Part model, mm, in its own coordinate system. A direction names the side the tool comes from. Round coordinates to 2 decimals unless told otherwise and drop trailing zeros. Write each loop counter-clockwise with the first axis right and the second up, starting at its lowest first coordinate (ties: lowest second). Pieces come first, ordered by that corner, then holes. Notation, with made-up numbers: (72.5, 68) -> (110.5, 68) arc R20 cw to (110.5, 93) -> close; hole circle Ø5 at (86, 8.25). An arc over 180 degrees is marked (long way). Use CSV: the item, a comma, the result in double quotes. Start each with the question number.
(1) Two-plate mould, pull along X, no slides. Class faces 1 (the flat face through (28, -14.05, -3)), 2 (the flat face through (21, 0, 6.5)), 3 (the flat face through (19.117, -16.704, 2.958)), 4 (the flat face through (29.408, -13, -1)): released by +X, released by -X, zero draft, split by the parting line, or undercut.
(2) Saw through at C-C (x = 10.5). Give the cut face in (y, z).
(3) Drop flat-ended pins along their axis: pin 1 (1.3 mm diameter, centred on x = 8, y = -17.5, fed in from -Z); pin 2 (1.9 mm diameter, centred on y = -22.5, z = 1.5, fed in from -X); pin 3 (0.6 mm diameter, centred on x = -26, z = -2.5, fed in from +Y); pin 4 (1.6 mm diameter, centred on y = 15, z = -1, fed in from +X). Give the stop position or say it passes through.
(4) Saw through at B-B (z = 1.25). Count the separate pieces of the cut face and the enclosed holes in it, plus the area to 3 significant figures.
(5) Saw through at A-A (y = 0). Give the cut face in (x, z), plus the area to 3 significant figures.
(6) Probe line 1 (Y direction, x = -23, z = 0.75); line 2 (X direction, y = 19.79, z = 4.75) (3 decimals); line 3 (Y direction, x = 12, z = 6.25). List the from-to ranges inside material, lowest first. Write a range as [from, to].
(7) Which spindle directions (+Z, -Z, +X, -X, +Y, -Y) get a long thin tool onto all of the face, cutting with end or side? Do faces 5 (the flat face through (24.908, 0, 3)), 6 (the flat face through (-5, -23, 2)), 7 (the cylindrical face through (-25.1, -13, -2.7)), 8 (the cylindrical face through (8.29, -16.61, 5.01)). Say none if no direction does.
```python
from build123d import *

# Parameters (mm, degrees)
PAD_DEPTH       = 6.5
POCKET_DEPTH    = 6
SKETCH002_R     = 13.5
POCKET001_DEPTH = 1
SKETCH003_W     = 5.4
SKETCH003_H     = 6.5
PAD001_DEPTH    = 4.5
POCKET002_DEPTH = 10
SKETCH010_W     = 3.95
SKETCH010_H     = 6.5
PAD002_DEPTH    = 4.5
POCKET005_DEPTH = 10
SKETCH014_R     = 20.45
SKETCH014_R_2   = 19.5
POCKET008_DEPTH = 0.3
SKETCH015_R     = 2.2
SKETCH015_R_2   = 0.975
PAD003_DEPTH    = 2
POCKET009_DEPTH = 4
POCKET010_DEPTH = 4
PAD004_DEPTH    = 4
SKETCH019_R     = 0.6
POCKET011_DEPTH = 2
SKETCH020_R     = 0.6
POCKET012_DEPTH = 2
FILLET_R        = 4
CHAMFER_SIZE    = 2.5
FILLET001_R     = 5


with BuildPart() as part:
    # Sketch → Pad (new body)
    with BuildSketch(Plane.XY):
        with BuildLine():
            Line((-22.5019915649, 16), (-22.5019915649, -16))
            Line((-22.5019915649, -16), (-16.2858834577, -17.9000000001))
            ThreePointArc((-16.2858834577, -17.9000000001), (0.2206895737, -24.1989937004), (16.6096357576, -17.5999999999))
            Line((16.6096357576, -17.5999999999), (24.9082802252, -17.45))
            Line((24.9082802252, 17.45), (24.9082802252, -17.45))
            Line((16.6096357576, 17.6), (24.9082802252, 17.45))
            ThreePointArc((16.6096357576, 17.6), (0.2206895736, 24.1989937004), (-16.2858834578, 17.9))
            Line((-22.5019915649, 16), (-16.2858834578, 17.9))
        make_face()
    extrude(amount=PAD_DEPTH)

    # Sketch001 → Pocket (cut)
    with BuildSketch(Plane.XY):
        with BuildLine():
            Line((-14.8539557021, 16.9), (-21.2122180433, 15.55))
            Line((-21.2122180433, 15.55), (-21.2122180433, -15.55))
            Line((-21.2122180433, -15.55), (-14.8539557021, -16.9))
            ThreePointArc((-14.8539557021, -16.9), (-0.0760301383, -22.4998715423), (14.739402973, -17))
            Line((14.739402973, -17), (23.6191552218, -16.4))
            Line((23.6191552218, 16.4), (23.6191552218, -16.4))
            Line((14.739402973, 17), (23.6191552218, 16.4))
            ThreePointArc((14.739402973, 17), (-0.0760301383, 22.4998715423), (-14.8539557021, 16.9))
        make_face()
    extrude(amount=POCKET_DEPTH, mode=Mode.SUBTRACT)

    # Sketch002 (on Face19 of Pocket) → Pocket001 (cut)
    with BuildSketch(Plane(origin=(0, 0, 6), x_dir=(1, 0, 0), z_dir=(0, 0, -1))):
        Circle(SKETCH002_R)
    extrude(amount=-POCKET001_DEPTH, mode=Mode.SUBTRACT)

    # Sketch003 (on Face7 of Pad) → Pad001 (join)
    with BuildSketch(Plane.YZ.offset(24.9082802252)):
        with Locations((-14.75, 3.25)):
            Rectangle(SKETCH003_W, SKETCH003_H)
        with Locations((14.75, 3.25)):
            Rectangle(SKETCH003_W, SKETCH003_H)
    extrude(amount=PAD001_DEPTH)

    # Sketch006 (on Face22 of Pad001) → Pocket002 (cut)
    with BuildSketch(Plane.XY.offset(6.5)):
        with BuildLine():
            ThreePointArc((24.9082802252, 17.45), (26.9423471239, 15.7065020586), (29.4082802252, 14.6594169811))
            Line((29.4082802252, 17.45), (29.4082802252, 14.6594169811))
            Line((29.4082802252, 17.45), (24.9082802252, 17.45))
        make_face()
        with BuildLine():
            ThreePointArc((29.4082802252, -14.6594169811), (26.9423471239, -15.7065020586), (24.9082802252, -17.45))
            Line((29.4082802252, -17.45), (24.9082802252, -17.45))
            Line((29.4082802252, -14.6594169811), (29.4082802252, -17.45))
        make_face()
    extrude(amount=-POCKET002_DEPTH, mode=Mode.SUBTRACT)

    # Sketch010 (on Face3 of Pad) → Pad002 (join)
    with BuildSketch(Plane(origin=(-22.5019915649, 0, 0), x_dir=(0, -1, 0), z_dir=(-1, 0, 0))):
        with Locations((-14.025, 3.25)):
            Rectangle(SKETCH010_W, SKETCH010_H)
        with Locations((14.025, 3.25)):
            Rectangle(SKETCH010_W, SKETCH010_H)
    extrude(amount=PAD002_DEPTH)

    # Sketch011 (on Face28 of Pad002) → Pocket005 (cut)
    with BuildSketch(Plane.XY.offset(6.5)):
        Polygon((-27.0019915649, 16), (-22.5019915649, 16), (-27.0019915649, 14.5), align=None)
        Polygon((-22.5019915649, -16), (-27.0019915649, -14.5), (-27.0019915649, -16), align=None)
    extrude(amount=-POCKET005_DEPTH, mode=Mode.SUBTRACT)

    # Sketch014 (on Face10 of Pad) → Pocket008 (cut)
    with BuildSketch(Plane.XY.offset(6.5)):
        Circle(SKETCH014_R)
        Circle(SKETCH014_R_2, mode=Mode.SUBTRACT)
    extrude(amount=-POCKET008_DEPTH, mode=Mode.SUBTRACT)

    # Sketch015 (on Face19 of Pocket) → Pad003 (join)
    with BuildSketch(Plane(origin=(0, 0, 6), x_dir=(1, 0, 0), z_dir=(0, 0, -1))):
        with Locations((-18.42, 13.32)):
            Circle(SKETCH015_R)
        with Locations((-18.42, 13.32)):
            Circle(SKETCH015_R_2, mode=Mode.SUBTRACT)
        with Locations((7.27, 18.56)):
            Circle(SKETCH015_R)
        with Locations((7.27, 18.56)):
            Circle(SKETCH015_R_2, mode=Mode.SUBTRACT)
        with Locations((5.37, -19.79)):
            Circle(SKETCH015_R)
        with Locations((5.37, -19.79)):
            Circle(SKETCH015_R_2, mode=Mode.SUBTRACT)
        with Locations((-18.42, -13.32)):
            Circle(SKETCH015_R)
        with Locations((-18.42, -13.32)):
            Circle(SKETCH015_R_2, mode=Mode.SUBTRACT)
    extrude(amount=PAD003_DEPTH)

    # Sketch016 → Pocket009 (cut)
    with BuildSketch(Plane(origin=(0, 0, 0), x_dir=(-1, 0, 0), z_dir=(0, 0, 1))):
        with BuildLine():
            Line((-5, 23.6778377391), (-5, 21.9374109685))
            ThreePointArc((5, 21.9374109685), (0, 22.5), (-5, 21.9374109685))
            Line((5, 23.6778377391), (5, 21.9374109685))
            ThreePointArc((5, 23.6778377391), (0, 24.2), (-5, 23.6778377391))
        make_face()
    extrude(amount=POCKET009_DEPTH, mode=Mode.SUBTRACT)

    # Sketch017 → Pocket010 (cut)
    with BuildSketch(Plane(origin=(0, 0, 0), x_dir=(-1, 0, 0), z_dir=(0, 0, 1))):
        with BuildLine():
            Line((-3.499984119, -22.2261132717), (-3.5, -23.9455632634))
            ThreePointArc((-3.5, -23.9455632634), (0, -24.2000019575), (3.5, -23.9455632634))
            Line((3.5000158811, -22.2261082701), (3.5, -23.9455632634))
            ThreePointArc((-3.499984119, -22.2261132717), (1.60767e-05, -22.5), (3.5000158811, -22.2261082701))
        make_face()
        with BuildLine():
            ThreePointArc((-13.9498796389, -17.6536358312), (-11.25, -19.4855715851), (-8.3135572795, -20.9077680626))
            Line((-8.3135572795, -20.9077680626), (-8.9416927184, -22.487466094))
            ThreePointArc((-15.0038705449, -18.987466094), (-12.1, -20.9578147716), (-8.9416927184, -22.487466094))
            Line((-13.9498796389, -17.6536358312), (-15.0038705449, -18.987466094))
        make_face()
        with BuildLine():
            ThreePointArc((8.3135572795, -20.9077680626), (11.25, -19.4855715851), (13.9498796389, -17.6536358312))
            Line((13.9498796389, -17.6536358312), (15.0038705449, -18.987466094))
            ThreePointArc((8.9416927184, -22.487466094), (12.1, -20.9578147716), (15.0038705449, -18.987466094))
            Line((8.3135572795, -20.9077680626), (8.9416927184, -22.487466094))
        make_face()
    extrude(amount=POCKET010_DEPTH, mode=Mode.SUBTRACT)

    # Sketch018 (on Face8 of Pocket005) → Pad004 (join)
    with BuildSketch(Plane(origin=(0, 0, 0), x_dir=(1, 0, 0), z_dir=(0, 0, -1))):
        Polygon((-27.0019915649, 14.5), (-27.0019915649, 12.05), (-22.5019915649, 12.05), (-22.5019915649, 16), align=None)
        Polygon((-27.0019915649, -12.05), (-22.5019915649, -12.05), (-22.5019915649, -16), (-27.0019915649, -14.5), align=None)
        with BuildLine():
            Line((24.9082802252, 17.45), (24.9082802252, 12.05))
            Line((29.4082802252, 12.05), (24.9082802252, 12.05))
            Line((29.4082802252, 14.6594169811), (29.4082802252, 12.05))
            ThreePointArc((24.9082802252, 17.45), (26.9423471239, 15.7065020586), (29.4082802252, 14.6594169811))
        make_face()
        with BuildLine():
            Line((24.9082802252, -12.05), (24.9082802252, -17.45))
            ThreePointArc((29.4082802252, -14.6594169811), (26.9423471239, -15.7065020586), (24.9082802252, -17.45))
            Line((29.4082802252, -12.05), (29.4082802252, -14.6594169811))
            Line((24.9082802252, -12.05), (29.4082802252, -12.05))
        make_face()
    extrude(amount=PAD004_DEPTH)

    # Sketch019 (on Face64 of Pad004) → Pocket011 (cut)
    with BuildSketch(Plane.XZ.offset(-12.05)):
        with Locations((28.1082802252, -2.7)):
            Circle(SKETCH019_R)
        with Locations((-25.7019915649, -2.7)):
            Circle(SKETCH019_R)
    extrude(amount=-POCKET011_DEPTH, mode=Mode.SUBTRACT)

    # Sketch020 (on Face50 of Pocket011) → Pocket012 (cut)
    with BuildSketch(Plane(origin=(0, -12.05, 0), x_dir=(-1, 0, 0), z_dir=(0, 1, 0))):
        with Locations((-28.1082802252, -2.7)):
            Circle(SKETCH020_R)
        with Locations((25.7019915649, -2.7)):
            Circle(SKETCH020_R)
    extrude(amount=-POCKET012_DEPTH, mode=Mode.SUBTRACT)

    # Fillet
    fillet_edges = [part.edges().sort_by_distance(p)[0] for p in [
        (29.40828, -13.354708, 6.5),
        (29.40828, 13.354708, 6.5),
        (-27.001992, -13.275, 6.5),
        (-27.001992, 13.275, 6.5),
    ]]
    fillet(fillet_edges, radius=FILLET_R)

    # Chamfer
    chamfer_edges = [part.edges().sort_by_distance(p)[0] for p in [
        (24.90828, -14.75, -4),
        (24.90828, 14.75, -4),
        (-22.501992, -14.025, -4),
        (-22.501992, 14.025, -4),
    ]]
    chamfer(chamfer_edges, length=CHAMFER_SIZE)

    # Fillet001
    fillet001_edges = [part.edges().sort_by_distance(p)[0] for p in [
        (16.609636, -17.6, 3.25),
        (-16.285883, -17.9, 3.25),
        (16.609636, 17.6, 3.25),
        (-16.285883, 17.9, 3.25),
    ]]
    fillet(fillet001_edges, radius=FILLET001_R)


solid = part.part
```
Answers:
1,face 1,"undercut"
1,face 2,"zero draft"
1,face 3,"undercut"
1,face 4,"released by +X"
2,outline,"(-21.8, 0) -> (-19.9, 0) -> (-19.9, 6) -> (-8.49, 6) -> (-8.49, 6.5) -> (-16.43, 6.5) -> (-16.43, 6.2) -> (-17.55, 6.2) -> (-17.55, 6.5) -> (-21.8, 6.5) -> close; (8.49, 6) -> (19.9, 6) -> (19.9, 4) -> (21.8, 4) -> (21.8, 6.5) -> (17.55, 6.5) -> (17.55, 6.2) -> (16.43, 6.2) -> (16.43, 6.5) -> (8.49, 6.5) -> close"
3,pin 1,"stops at z = 4"
3,pin 2,"stops at x = -11.01"
3,pin 3,"stops at y = 14.93"
3,pin 4,"stops at x = 29.41"
4,separate pieces,"4"
4,enclosed holes,"0"
4,area,"240 mm²"
5,outline,"(-22.5, 0) -> (-21.21, 0) -> (-21.21, 6) -> (-13.5, 6) -> (-13.5, 6.5) -> (-19.5, 6.5) -> (-19.5, 6.2) -> (-20.45, 6.2) -> (-20.45, 6.5) -> (-22.5, 6.5) -> close; (13.5, 6) -> (23.62, 6) -> (23.62, 0) -> (24.91, 0) -> (24.91, 6.5) -> (20.45, 6.5) -> (20.45, 6.2) -> (19.5, 6.2) -> (19.5, 6.5) -> (13.5, 6.5) -> close"
5,area,"25.1 mm²"
6,line 1,"y = [-15.83, -12.05], [12.05, 15.83]"
6,line 2,"x = [-13.928, -10.705], [3.17, 4.395], [6.345, 7.57], [10.705, 13.928]"
6,line 3,"y = [-21.02, -16.56], [-15.37, -6.18], [6.18, 15.37], [16.56, 21.02]"
7,face 5,"+Z, -Z, +X"
7,face 6,"-Z, -Y"
7,face 7,"none"
7,face 8,"-Z"
